The model under review builds one solid part; all positions refer to its coordinate system, in mm. A direction names the side the tool comes from. Give positions to 0.01 mm unless a question says otherwise; leave off trailing zeros. Write item = value, one per line. Start each with the question number.
1. Wall thickness on line 1 along Z through (x, y) = (-246, 295.5); line 2 along Z through (x, y) = (-287.5, 279.5); line 3 along X through (y, z) = (387, -135): over which ranges is each line inside the solid? List them lowest first. Write a range as from..to.
2. For faces 1 (the face through (8.302, 621, -172)), 2 (the face through (8.302, 621, 172)), 3 (the face through (-16, 362, 237.5)), list the 3-axis set-ups (+Z, -Z, +X, -X, +Y, -Y) from which the entire face can be reached by the end or side of a thin tool; tool diameter is ignored.
3. For pin 1 (8 mm diameter, centred on y = 399.5, z = 81.5, fed in from -X); pin 2 (3 mm diameter, centred on y = 651.5, z = 104, fed in from +X); pin 3 (3 mm diameter, centred on x = 23, z = 2, fed in from +Y), all flat-tipped, find the tip position at first contact; note any pin that passes through.
from build123d import *

# Parameters (mm, degrees)
BOSS_EXTRUDE1_DEPTH          = 237.5
BOSS_EXTRUDE1_DEPTH_BACK     = 237.5
SKETCH1_RX                   = 712.26718515
SKETCH1_RY                   = 343.28059296
SKETCH7_W                    = 1048.477934303
SKETCH7_H                    = 944.198935412
CUT_EXTRUDE2_DEPTH           = 923.383384794
CUT_REVOLVE4_ANGLE           = 90
CUT_REVOLVE4_OTHER_WAY_ANGLE = 90


with BuildPart() as part:
    # Sketch1 → Boss-Extrude1 (new, two sides: drawn at the far end of the back side and taken through both)
    with BuildSketch(Plane.XY.offset(-BOSS_EXTRUDE1_DEPTH_BACK)):
        with Locations(Location((0, 0), (0, 0, 90))):
            Ellipse(SKETCH1_RX, SKETCH1_RY)
    extrude(amount=BOSS_EXTRUDE1_DEPTH + BOSS_EXTRUDE1_DEPTH_BACK)

    # Sketch7 → Cut-Extrude2 (cut, through all)
    with BuildSketch(Plane.XY.offset(237.5)):
        with Locations((-29.38771787, -262.502282556)):
            Rectangle(SKETCH7_W, SKETCH7_H)
    extrude(amount=-CUT_EXTRUDE2_DEPTH, mode=Mode.SUBTRACT)

    # Sketch11 → Cut-Revolve2 (revolve, cut)
    with BuildSketch(Plane.XY):
        with BuildLine():
            Line((-343.28059296, 0), (-743.226651757, 0))
            Line((-743.226651757, 0), (-743.226651757, 860.341056905))
            Line((-743.226651757, 860.341056905), (0, 860.341056905))
            Line((0, 860.341056905), (0, 712.26718515))
            add(Edge.make_bspline(
                [(0, 712.26718515), (-343.28059296, 712.26718515), (-343.28059296, 0)],
                knots=[0, 0, 0, 1.570796327, 1.570796327, 1.570796327], degree=2, weights=[1, 0.707106781, 1]))
        make_face()
    revolve(axis=Axis((65.79623911, 0, 0), (0, 1, 0)), mode=Mode.SUBTRACT)

    # Sketch15 → Cut-Revolve4 (revolve, cut)
    with BuildSketch(Plane.XY):
        with BuildLine():
            Line((8.302449854, 946.581815565), (524.826005951, 946.581815565))
            Line((524.826005951, 946.581815565), (524.826005951, 209.59718515))
            Line((524.826005951, 209.59718515), (328.081176474, 209.597185149))
            add(Edge.make_bspline(
                [(328.081176474, 209.597185149), (255.359120318, 699.657333261), (8.302449854, 712.0588366)],
                knots=[5.011078122, 5.011078122, 5.011078122, 6.258997341, 6.258997341, 6.258997341], degree=2, weights=[1, 0.81157141, 1]))
            Line((8.302449854, 712.0588366), (8.302449854, 946.581815565))
        make_face()
    revolve(axis=Axis((8.302449854, 1026.356298718, 0), (0, 1, 0)), revolution_arc=CUT_REVOLVE4_ANGLE, mode=Mode.SUBTRACT)

    # Sketch15 → Cut-Revolve4 other way (revolve, cut)
    with BuildSketch(Plane.XY):
        with BuildLine():
            Line((8.302449854, 946.581815565), (524.826005951, 946.581815565))
            Line((524.826005951, 946.581815565), (524.826005951, 209.59718515))
            Line((524.826005951, 209.59718515), (328.081176474, 209.597185149))
            add(Edge.make_bspline(
                [(328.081176474, 209.597185149), (255.359120318, 699.657333261), (8.302449854, 712.0588366)],
                knots=[5.011078122, 5.011078122, 5.011078122, 6.258997341, 6.258997341, 6.258997341], degree=2, weights=[1, 0.81157141, 1]))
            Line((8.302449854, 712.0588366), (8.302449854, 946.581815565))
        make_face()
    revolve(axis=Axis((8.302449854, 1026.356298718, 0), (0, -1, 0)), revolution_arc=CUT_REVOLVE4_OTHER_WAY_ANGLE, mode=Mode.SUBTRACT)


solid = part.part
Final values:
q1.line_1 = -213.95..213.95
q1.line_2 = -144.07..144.07
q1.line_3 = -261.44..253.48
q2.face_1 = -Z, +X, +Y
q2.face_2 = +Z, +X, +Y
q2.face_3 = +Z, +X, -X, +Y, -Y
q3.pin_1 = -276.21
q3.pin_2 = 90.32
q3.pin_3 = 710.85
